Part model, mm, in its own coordinate system. Coordinates: 2 decimals unless noted, no trailing zeros. Loops run counter-clockwise (first coordinate to the right, second up) from the corner with the lowest first, then second, coordinate; pieces in that order, holes last. Notation, with made-up numbers: M 35.25,72 L 76.25,72 A27 ccw 76.25,94 Z; hole C 10.5,33 d8. An arc over 180 degrees is marked long. Use a Markdown table: item, result. Add a question column.
1) Band-saw the part on A-A (x = 519). List the corners of the cut face in (y, z), plus the area to 3 significant figures.
2) Wall check: probe 1 along Y at (x, z) = (495.5, 0.75); probe 2 along Z at (x, y) = (48, -0.5); probe 3 along X at (y, z) = (4.75, 1.5). Give the ranges that are in metal, low to high. Write a range as from..to.
3) Pin check, flat tips, straight feed: pin 1 Ø2 at (y, z) = (-0.5, 3) entering from -X; pin 2 Ø6 at (y, z) = (-3.5, 2.5) entering from +X; pin 3 Ø6 at (y, z) = (-2, 2) entering from +X; pin 4 Ø1.8 at (x, y) = (393, 0.5) entering from +Z. Stop position of each tip, or through.
4) Band-saw the part on B-B (z = -1). List the corners of the cut face in (x, y).
from build123d import *

# Parameters (mm, degrees)
F1_DEPTH   = 704
F2_C1_SIZE = 9.9999
F2_C2_SIZE = 9.9999


# Not quite as in the source:
# - a fillet or chamfer is up to 0.001 mm smaller than in the source, because OpenCascade refuses the exact size


with BuildPart() as f1:
    # F0 (on Right) → F1 (new body)
    with BuildSketch(Plane.YZ):
        Polygon((-3, 5), (-5, 5), (-5, -5), (5, -5), (5, 5), (3, 5), (3, -3), (-3, -3), align=None)
    extrude(amount=F1_DEPTH)

    # F2: chamfer of 10 on 3 edges, made by hand

    # F2_c1 (size 10 in the source; OpenCascade refuses exactly that, so slightly less here)
    f2_c1_edges = [f1.edges().sort_by_distance(p)[0] for p in [
        (0, -4, 5),
    ]]
    chamfer(f2_c1_edges, length=F2_C1_SIZE)

    # F2_c2 (size 10 in the source; OpenCascade refuses exactly that, so slightly less here)
    f2_c2_edges = [f1.edges().sort_by_distance(p)[0] for p in [
        (704, -4, 5),
    ]]
    chamfer(f2_c2_edges, length=F2_C2_SIZE)


solid = f1.part
Entries:
| question | item | result |
|---|---|---|
| 1 | outline | M -5,-5 L 5,-5 L 5,5 L 3,5 L 3,-3 L -3,-3 L -3,5 L -5,5 Z |
| 1 | area | 52.0 mm2 |
| 2 | probe 1 | -5..-3, 3..5 |
| 2 | probe 2 | -5..-3 |
| 2 | probe 3 | 6.5..697.5 |
| 3 | pin 1 | through |
| 3 | pin 2 | x = 699.5 |
| 3 | pin 3 | x = 699.83 |
| 3 | pin 4 | z = -3 |
| 4 | outline | M 4,-5 L 700,-5 L 700,-3 L 4,-3 Z; M 4,3 L 700,3 L 700,5 L 4,5 Z |
